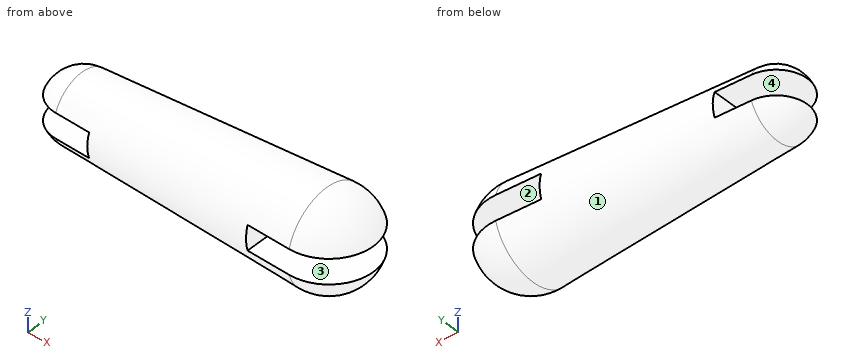
```python
from build123d import *

# Parameters (mm, degrees)
CUT_EXTRUDE1_DEPTH      = 186.063012512
CUT_EXTRUDE1_DEPTH_BACK = 186.063012512
SKETCH4_W               = 93.98
SKETCH4_H               = 25.4
SKETCH4_W_2             = 68.58


with BuildPart() as part:
    # Sketch3 → Revolve2 (revolve)
    with BuildSketch(Plane(origin=(0, 0, 0), x_dir=(1, 0, 0), z_dir=(0, 1, 0))):
        with BuildLine():
            Line((-125.73, 0), (125.73, 0))
            Line((125.73, 0), (172.72, 0))
            ThreePointArc((172.72, 0), (158.10701278, 34.05567711), (123.356767677, 46.930031625))
            Line((123.356767677, 46.930031625), (-127.461818182, 34.246239294))
            ThreePointArc((-127.461818182, 34.246239294), (-150.581440053, 23.626468786), (-160.02, 0))
            Line((-160.02, 0), (-125.73, 0))
        make_face()
    revolve(axis=Axis((-1000, 0, 0), (1, 0, 0)))

    # Sketch4 → Cut-Extrude1 (cut, two sides: drawn at the far end of the back side and taken through both)
    with BuildSketch(Plane(origin=(0, 0, 0), x_dir=(1, 0, 0), z_dir=(0, 1, 0)).offset(-CUT_EXTRUDE1_DEPTH_BACK)):
        with Locations((125.73, 0)):
            Rectangle(SKETCH4_W, SKETCH4_H)
        with Locations((-125.73, 0)):
            Rectangle(SKETCH4_W_2, SKETCH4_H)
    extrude(amount=CUT_EXTRUDE1_DEPTH + CUT_EXTRUDE1_DEPTH_BACK, mode=Mode.SUBTRACT)


solid = part.part
```
Read the model definition and answer for the solid it produces. Units are mm, in the model's axes. Face numbers are marked on the shaded views. A direction names the side the tool comes from. Give positions to 0.01 mm unless a question says otherwise; leave off trailing zeros. Order: outer loops, then holes, each group sorted by start corner. A loop starts at its lowest first (then second) coordinate and runs counter-clockwise, first axis right, second up.
(1) Straight lines are drawn through the part: L1, parallel to X at y = 9.5, z = -11; L2, parallel to Y at x = -80, z = -13; L3, parallel to Z at x = -105, y = -26.5. For each, find the intervals that lie inside material, in ascending order.
(2) Find section D-D (x = -52.5). Give the vertices of the cut face in (y, z).
(3) Find section C-C (z = 0). Give the vertices of the cut face in (x, y), plus the area to 3 significant figures.
(4) Find section B-B (x = 132). Give the vertices of the cut face in (y, z).
(5) For a pull along Z with two mould halves and no side action, classify the marked faces 1 and 2 as released by +Z, released by -Z, zero draft, split by the parting line, or undercut.
(6) Find section A-A (y = 0). Give the vertices of the cut face in (x, z).
(7) Given pin 1 (2 mm diameter, centred on x = 126.5, y = -12.5, fed in from -Z); pin 2 (7.5 mm diameter, centred on y = 5, z = -3, fed in from -X); pin 3 (2 mm diameter, centred on x = 37, y = 4.5, fed in from -Z), each flat-ended and moving along its own axis, determine where each tip first touches the part or whether it passes through.
(8) For the marked faces 3 and 4, determine the directions among +Z, -Z, +X, -X, +Y, -Y from which every point of the face is accessible in a straight line to the end or side of a thin tool.
Result sheet:
1. L1: x = -91.44 to 78.74
1. L2: y = -34.26 to 34.26
1. L3: z = -23.44 to -12.7, 12.7 to 23.44
2. outline: circle Ø76.07 at (0, 0)
3. outline: (-91.44, -36.07) - (78.74, -44.67) - (78.74, 44.67) - (-91.44, 36.07) - close
3. area: 13,700 mm2
4. outline: (-44.8, -12.7) arc R46.57 ccw to (44.8, -12.7) - close; (-44.8, 12.7) - (44.8, 12.7) arc R46.57 ccw to start
5. face 1: split by the parting line
5. face 2: undercut
6. outline: (-157.58, -12.7) arc R34.29 ccw to (-127.46, -34.25) - (123.36, -46.93) arc R46.99 ccw to (170.97, -12.7) - (78.74, -12.7) - (78.74, 12.7) - (170.97, 12.7) arc R46.99 ccw to (123.36, 46.93) - (-127.46, 34.25) arc R34.29 ccw to (-157.58, 12.7) - (-91.44, 12.7) - (-91.44, -12.7) - close
7. pin 1: stops at z = -45.56
7. pin 2: stops at x = -91.44
7. pin 3: stops at z = -42.43
8. face 3: +X, +Y, -Y
8. face 4: -X, +Y, -Y
